Verification items for the finished model (mm, model axes). Face numbers are marked on the shaded views. A direction names the side the tool comes from. Round coordinates to 2 decimals unless told otherwise and drop trailing zeros. Loops run counter-clockwise (first coordinate to the right, second up) from the corner with the lowest first, then second, coordinate; pieces in that order, holes last.
from build123d import *

# Parameters (mm, degrees)
SKETCH2_R           = 11
BOSS_EXTRUDE1_DEPTH = 30
CUT_EXTRUDE1_DEPTH  = 70
BOSS_EXTRUDE3_DEPTH = 40
CUT_EXTRUDE2_DEPTH  = 46
FILLET1_R           = 15


with BuildPart() as part:
    # Sketch2 → Boss-Extrude1 (new body)
    with BuildSketch(Plane(origin=(0, 0, 0), x_dir=(1, 0, 0), z_dir=(0, 1, 0))):
        Polygon((-63.982218383188474, 1.2957443941801692), (-63.98221838318849, -23.70425560581983), (26.017781616811508, -23.70425560581983), (26.017781616811508, 46.295744394180176), (-28.982218383188492, 46.29574439418017), (-28.982218383188492, 1.2957443941801692), align=None)
        with Locations(Location((-3.9822183831884903, -5.704255605819837, 0), (0, 0, 270))):
            Circle(SKETCH2_R, mode=Mode.SUBTRACT)
        with Locations(Location((-3.9822183831884903, 28.295744394180172, 0), (0, 0, 270))):
            Circle(SKETCH2_R, mode=Mode.SUBTRACT)
    extrude(amount=BOSS_EXTRUDE1_DEPTH)

    # Sketch3 → Cut-Extrude1 (cut)
    with BuildSketch(Plane.XY.offset(23.70425560581983)):
        Polygon((-63.98221838318849, 0), (16.01778161681151, 0), (16.017781616811508, 8), (-28.982218383188492, 7.999999999999995), (-28.982218383188492, 12.999999999999995), (-63.982218383188496, 12.999999999999995), align=None)
    extrude(amount=-CUT_EXTRUDE1_DEPTH, mode=Mode.SUBTRACT)

    # 3DSketch1 → Boss-Extrude3 (add)
    with BuildSketch(Plane(origin=(-63.98221838318849, 12.999999999999995, -1.2957443941801692), x_dir=(0, 0.8969047134125312, 0.4422238517520119), z_dir=(-1, 0, 0))):
        Polygon((0, 0), (11.055596293800297, -22.422617835313282), (53.21011782418927, -1.6380968029687248), (57.85346826758539, -11.055596293800305), (80.27608610289867, 0), (76.73829528888258, 7.1752377073002505), (63.28472458769462, 0.5418799310200721), (50.018009035134256, 27.449021333396008), (63.47157973632223, 34.08237910967619), (59.93378892230613, 41.25761681697644), (37.511171086992846, 30.20202052317613), (42.15452153038897, 20.784521032344557), align=None)
    extrude(amount=BOSS_EXTRUDE3_DEPTH)

    # Sketch4 → Cut-Extrude2 (cut)
    with BuildSketch(Plane.XY.offset(23.70425560581983)):
        Polygon((-103.9822183831885, 12.999999999999993), (-78.9822183831885, 13), (-78.9822183831885, 60), (-103.9822183831885, 60), align=None)
    extrude(amount=-CUT_EXTRUDE2_DEPTH, mode=Mode.SUBTRACT)

    # Fillet1
    fillet1_edges = [part.edges().sort_by_distance(p)[0] for p in [
        (-78.9822183831885, 13, 11.204255605819831),
    ]]
    fillet(fillet1_edges, radius=FILLET1_R)


solid = part.part
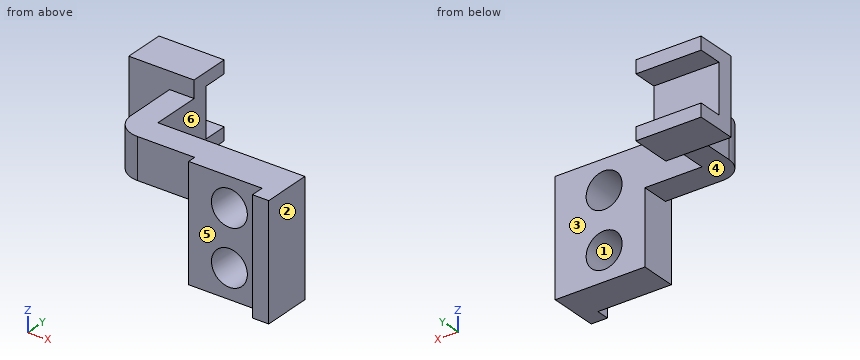
1. Gauge pin test, flat ends, axial feed: P1, Ø3, axis at y = 19, z = 5.5, coming from the -X side; P2, Ø1, axis at x = -28, z = -6.5, coming from the +Y side; P3, Ø3, axis at x = -27, z = -34, coming from the -Y side; P4, Ø10, axis at x = 0, z = 7, coming from the -Y side. Record the tip position at first contact, or that the pin passes through.
2. Section check B-B (z = -35). Enter the section's corners in (x, y).
3. Release check for a two-part mould opening along X. For the marked faces 1, 2 and 3 record: released by +X, released by -X, zero draft, split by the parting line, or undercut.
4. Section check C-C (x = -11). Enter the section's corners in (y, z).
5. Section check A-A (y = 77.5). Enter the section's corners in (x, z).
6. Tool access check on the marked faces 4, 5 and 6. Record the directions out of +Z, -Z, +X, -X, +Y, -Y that give a thin tool (end or side, any length) a straight path to the whole face; none if there is none.
7. Section check D-D (z = 21). Enter the section's corners in (x, y).
8. Scan lines: L1, parallel to X at y = 31, z = 6; L2, parallel to X at y = 73, z = -11.5; L3, parallel to Z at x = -69, y = 36.5. Record each from-to range of solid material in increasing order.
Taken from the geometry:
1. P1: stops at x = -76.97
1. P2: stops at y = 30
1. P3: stops at y = 8
1. P4: passes through
2. outline: (-28.98, 8) - (-12.7, 8) - (-12.7, 30) - (-28.98, 30) - close; (4.74, 8) - (16.02, 8) - (16.02, 0) - (26.02, 0) - (26.02, 30) - (4.74, 30) - close
3. face 1: undercut
3. face 2: released by +X
3. face 3: zero draft
4. outline: (8, -46.3) - (30, -46.3) - (30, -36.77) - (8, -36.77) - close; (8, -19.83) - (30, -19.83) - (30, -2.77) - (8, -2.77) - close; (8, 14.17) - (30, 14.17) - (30, 23.7) - (8, 23.7) - close
5. outline: (-103.98, -11.8) - (-63.98, -11.8) - (-63.98, -3.8) - (-103.98, -3.8) - close; (-103.98, 26.2) - (-63.98, 26.2) - (-63.98, 34.2) - (-103.98, 34.2) - close
6. face 4: -Z, -X, -Y
6. face 5: +Z, -Z, -X, -Y
6. face 6: +Z, -Z, +X, +Y
7. outline: (-103.98, 60) - (-78.98, 60) - (-78.98, 28) arc R15 ccw to (-63.98, 13) - (-28.98, 13) - (-28.98, 8) - (16.02, 8) - (16.02, 0) - (26.02, 0) - (26.02, 30) - (-63.98, 30) - (-63.98, 70) - (-103.98, 70) - close
8. L1: x = -78.98 to -63.98
8. L2: x = -103.98 to -63.98
8. L3: z = -1.3 to 23.7
